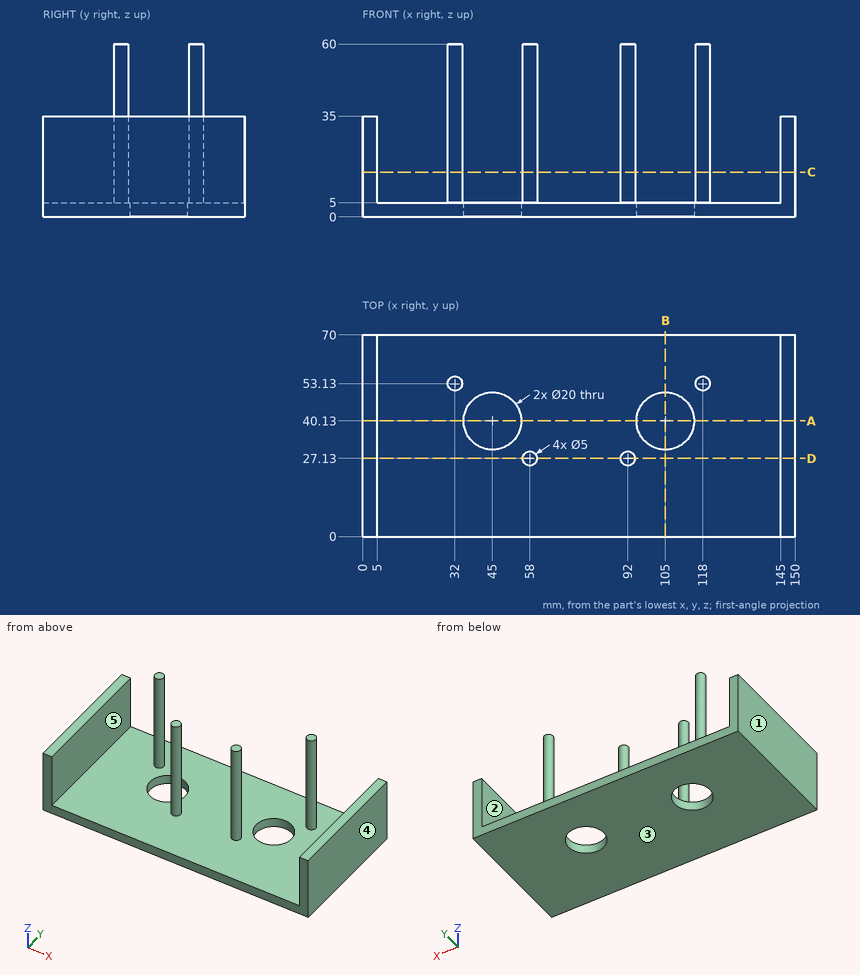
Could you check a few things on this drawing? It's one solid part, dimensions in mm from its lowest x, y, z. A direction names the side the tool comes from. Round coordinates to 2 decimals unless told otherwise and drop trailing zeros. Loops run counter-clockwise (first coordinate to the right, second up) from the corner with the lowest first, then second, coordinate; pieces in that order, holes last.
Q1. I want a section at D-D (y = 27.13). Write out the boundary of the cut face in (x, z), and give its area (3 significant figures).
Q2. On a 3-axis mill with a long thin cutter (end or side, diameter ignored), from which of +Z, -Z, +X, -X, +Y, -Y can I reach the whole of each face in a straight line? I mean the marked faces 4 and 5. Say none if no direction works.
Q3. I want a section at A-A (y = 40.13). Write out the boundary of the cut face in (x, z).
Q4. For P1, Ø18, axis at x = 45, y = 40.13, coming from the -Z side; P2, Ø2, axis at x = 89.5, y = 42.5, coming from the +Z side; P3, Ø4, axis at x = 56.5, z = 50.5, coming from the +Y side; P4, Ø4, axis at x = 3.5, y = 45.5, coming from the +Z side, each with a flat end and sliding along its axis, tell me the tip position at first contact or that it passes through.
Q5. I want a section at C-C (z = 15.5). Write out the boundary of the cut face in (x, y), and give its area (3 significant figures).
Q6. I want a section at B-B (x = 105). Write out the boundary of the cut face in (y, z).
Q7. Thinking about a two-plate mould opening in X: for the marked faces 1, 2 and 3, which applies, pulls with the +X half, pulls with the -X half, needs draft (parallel to the pull), parting line crosses it, or undercut?
Q8. Please list where these lines run through material, in increasing order: L1, parallel to X at y = 40, z = 3; L2, parallel to X at y = 30.5, z = 18.5; L3, parallel to Y at x = 45, z = 2.95.
Answer below:
1. outline: (0, 0) - (150, 0) - (150, 35) - (145, 35) - (145, 5) - (94.5, 5) - (94.5, 60) - (89.5, 60) - (89.5, 5) - (60.5, 5) - (60.5, 60) - (55.5, 60) - (55.5, 5) - (5, 5) - (5, 35) - (0, 35) - close
1. area: 1,600 mm2
2. face 4: +Z, -Z, +X, +Y, -Y
2. face 5: +Z, +Y, -Y
3. outline: (0, 0) - (35, 0) - (35, 5) - (5, 5) - (5, 35) - (0, 35) - close; (55, 0) - (95, 0) - (95, 5) - (55, 5) - close; (115, 0) - (150, 0) - (150, 35) - (145, 35) - (145, 5) - (115, 5) - close
4. P1: passes through
4. P2: stops at z = 5
4. P3: stops at y = 29.63
4. P4: stops at z = 35
5. outline: (0, 0) - (5, 0) - (5, 70) - (0, 70) - close; circle Ø5 at (32, 53.13); circle Ø5 at (58, 27.13); circle Ø5 at (92, 27.13); circle Ø5 at (118, 53.13); (145, 0) - (150, 0) - (150, 70) - (145, 70) - close
5. area: 779 mm2
6. outline: (0, 0) - (30.13, 0) - (30.13, 5) - (0, 5) - close; (50.13, 0) - (70, 0) - (70, 5) - (50.13, 5) - close
7. face 1: pulls with the -X half
7. face 2: undercut
7. face 3: needs draft
8. L1: x = 0 to 35, 55 to 95, 115 to 150
8. L2: x = 0 to 5, 145 to 150
8. L3: y = 0 to 30.13, 50.13 to 70
